Source: CAD feature listing. Evaluate the final solid. Frame: model axes, mm. A direction names the side the tool comes from. Coordinates: 2 decimals unless noted, no trailing zeros. Loops run counter-clockwise (first coordinate to the right, second up) from the corner with the lowest first, then second, coordinate; pieces in that order, holes last.
from build123d import *

# Parameters (mm, degrees)
SKETCH002_R     = 2.5
PAD001_DEPTH    = 15
CHAMFER001_SIZE = 1
PAD_DEPTH       = 2
CHAMFER_SIZE    = 0.25


with BuildPart() as body002:
    # Sketch002 → Pad001 (new body)
    with BuildSketch(Plane.XY):
        Circle(SKETCH002_R)
    extrude(amount=-PAD001_DEPTH)

    # Chamfer001
    chamfer001_edges = [body002.edges().sort_by_distance(p)[0] for p in [
        (-2.5, 0, -15),
    ]]
    chamfer(chamfer001_edges, length=CHAMFER001_SIZE)


with BuildPart() as body001:
    # Sketch001 → Pad (new body)
    with BuildSketch(Plane.XY):
        Polygon((1.5, -0.8660254038), (1.5, 0.8660254038), (0, 1.7320508076), (-1.5, 0.8660254038), (-1.5, -0.8660254038), (0, -1.7320508076), align=None)
    extrude(amount=PAD_DEPTH)


with BuildPart() as fusion:
    # Sketch → Revolution (revolve)
    with BuildSketch(Plane.XZ):
        with BuildLine():
            Line((0, -1.19), (4.75, -1.19))
            Line((4.75, -1.19), (4.75, -1.09))
            ThreePointArc((4.75, -1.09), (3.9738329701, 0.7838329701), (2.1, 1.56))
            Line((1.5, 1.56), (2.1, 1.56))
            Line((1.5, 0), (1.5, 1.56))
            Line((2.1, 0), (1.5, 0))
            Line((0, -1.19), (2.1, 0))
        make_face()
    revolve(axis=Axis((0, 0, 0), (0, 0, 1)))

    # Chamfer
    chamfer_edges = [fusion.edges().sort_by_distance(p)[0] for p in [
        (-1.5, 0, 1.56),
    ]]
    chamfer(chamfer_edges, length=CHAMFER_SIZE)

    # Cut: cut Body001
    add(body001.part, mode=Mode.SUBTRACT)


with BuildPart() as fusion_1:
    # Cut placement: moved
    add(fusion.part.moved(Location((0, 0, 1.19))))

    # Fusion: union Body002
    add(body002.part)


solid = fusion_1.part
Q1. Section A-A, the plane z = -1. Return the cut outline in (x, y), plus the area to 3 significant figures.
Q2. Line query: line 1 along Y through (x, z) = (0, -2.75); line 2 along X through (y, z) = (2.25, -6); line 3 along Z through (x, y) = (-1, -1.5). Output: solid intervals per line, ascending.
Q3. Contact query for flat-ended pins moving along their axis: pin 1 Ø0.8 at (y, z) = (0, 2) entering from +X; pin 2 Ø1.5 at (x, y) = (0.5, 2.5) entering from +Z; pin 3 Ø4 at (y, z) = (-2.5, -12.5) entering from +X; pin 4 Ø1 at (y, z) = (-1, -5.5) entering from -X. Output: stop coordinate, or through.
Q4. Draft query along Y for faces 1 (the cylindrical face through (-0.54, -2.44, -6.9)), 2 (the flat face through (1.5, 0, 2)), 3 (the flat face through (-2, -2, 0)). Return one class per face: +Y half, -Y half, draft (parallel to the pull), parting line (faces both ways), or undercut.
Q5. Access query for faces 4 (the conical face through (0, 0, 0)), 5 (the flat face through (0, 0, -15)), 6 (the flat face through (-1.5, 0, 2)). Directions: +Z, -Z, +X, -X, +Y, -Y. A direction counts if a zero-diameter tool reaches every point of the face in a straight line with its end or side. Return the directions, or none.
Derived:
1. outline: circle Ø5 at (0, 0)
1. area: 19.6 mm2
2. line 1: y = -2.5 to 2.5
2. line 2: x = -1.09 to 1.09
2. line 3: z = -14.7 to 1.02, 1.19 to 2.75
3. pin 1: stops at x = 4.28
3. pin 2: stops at z = 2.75
3. pin 3: stops at x = 2.45
3. pin 4: stops at x = -2.45
4. face 1: parting line
4. face 2: undercut
4. face 3: draft
5. face 4: none
5. face 5: -Z, +X, -X, +Y, -Y
5. face 6: +Z
